Autodesk Inventor part; units mm, degrees
ref_plane "YZ Plane" through (0, 0, 0) normal (1, 0, 0) x (0, 1, 0)
ref_plane "XZ Plane" through (0, 0, 0) normal (0, 1, 0) x (-1, 0, 0)
ref_plane "XY Plane" through (0, 0, 0) normal (0, 0, 1) x (1, 0, 0)
sketch "スケッチ1" plane through (0, 0, 0) normal (0, 0, 1) x (1, 0, 0)
  line L0 (0, 0) -> (5, 0)
  line L1 (5, 0) -> (5, 5)
  line L2 (5, 5) -> (0, 5)
  line L3 (0, 5) -> (0, 0)
  dimension "d0" = 5
  dimension "d1" = 5
extrude "押し出し1" add sketch "スケッチ1" along normal blind 80
sketch "スケッチ2" plane through (0, 0, 80) normal (0, 0, 1) x (1, 0, 0)
  line L0 (0, 0) -> (5, 0)
  line L1 (0, 5) -> (0, 0)
  point P0 (2.5, 2.5)
  point P1 (2.5, 0)
  point P2 (0, 2.5)
hole "穴1" at (2.5, 2.5, 80) direction (0, 0, -1) diameter 2.459 depth 8.8 tip angle 118
sketch "スケッチ3" plane through (0, 0, 0) normal (0, 0, -1) x (-1, 0, 0)
  line L0 (0, 5) -> (0, 0)
  line L1 (-5, 5) -> (0, 5)
  point P0 (-2.5, 2.5)
  point P1 (0, 2.5)
  point P2 (-2.5, 5)
hole "穴2" at (2.5, 2.5, 0) direction (0, 0, 1) diameter 2.459 depth 8.8 tip angle 118
properties part number "天板スペーサ"
Read the model definition and answer for the solid it produces. Units are mm, in the model's axes. A direction names the side the tool comes from. Coordinates: 2 decimals unless noted, no trailing zeros. Write each loop counter-clockwise with the first axis right and the second up, starting at its lowest first coordinate (ties: lowest second). Pieces come first, ordered by that corner, then holes. Notation, with made-up numbers: (-26.5, -31.5) - (26.5, -31.5) arc R18 cw to (26.5, -4.5) - close; hole circle Ø2 at (15, 10.5). An arc over 180 degrees is marked (long way). Answer as a JSON object with one key per item and string values. Group by question number.
1. The mould has two halves that part along Y. Classify faces 1 (the flat face through (2, 4, 0)), 2 (the flat face through (3, 5, 39)), 3 (the conical face through (2.29, 2.55, 70.59)): +Y half, -Y half, draft (parallel to the pull), parting line (faces both ways), or undercut.
2. Consider L1, parallel to Y at x = 2.5, z = 6.25; L2, parallel to Y at x = 1.4, z = 7.5. Determine where each line is inside the solid, lowest interval first. Write a range as [from, to].
3. This flat-tipped pin is pushed along its axis until it touches: P1, Ø2, axis at x = 2.5, y = 2.5, coming from the +Z side. Where does it stop, or does it pass through?
4. Which of the six approach directions +Z, -Z, +X, -X, +Y, -Y give full straight-line access (tool end or side, diameter ignored) to faces 4 (the cylindrical face through (2.131, 3.673, 4.462)), 5 (the cylindrical face through (2.131, 1.327, 75.538)), 6 (the flat face through (0, 3, 39))?
5. A cutting plane is placed at A-A (z = 74). Determine the outline of the cut face in (x, y), plus the area to 3 significant figures.
Worked out:
{
 "1": {"face 1": "draft", "face 2": "+Y half", "face 3": "undercut"},
 "2": {"L1": "y = [0, 1.27], [3.73, 5]", "L2": "y = [0, 1.95], [3.05, 5]"},
 "3": {"P1": "stops at z = 71.06"},
 "4": {"face 4": "-Z", "face 5": "+Z", "face 6": "+Z, -Z, -X, +Y, -Y"},
 "5": {"outline": "(0, 0) - (5, 0) - (5, 5) - (0, 5) - close; hole circle Ø2.46 at (2.5, 2.5)", "area": "20.3 mm²"}
}
